Model file for the job. Use its own axes, mm. Round coordinates to 2 decimals unless told otherwise and drop trailing zeros. Use one line per item in the form item = value.
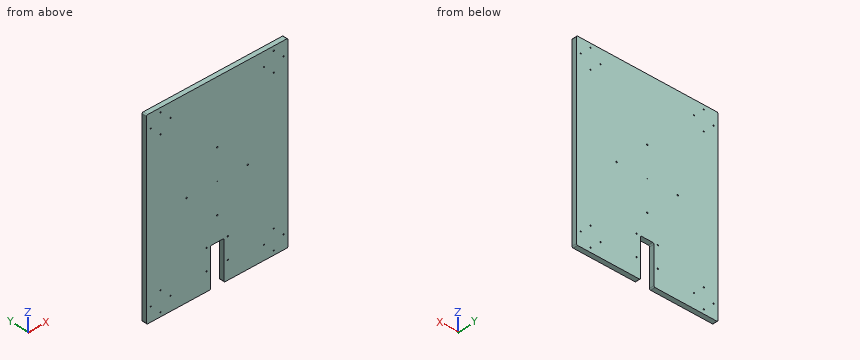
Autodesk Inventor part; units mm, degrees
ref_plane "YZ Plane" through (0, 0, 0) normal (1, 0, 0) x (0, 1, 0)
ref_plane "XZ Plane" through (0, 0, 0) normal (0, 1, 0) x (-1, 0, 0)
ref_plane "XY Plane" through (0, 0, 0) normal (0, 0, 1) x (1, 0, 0)
sketch "Sketch1" plane through (0, 0, 0) normal (0, 1, 0) x (-1, 0, 0)
  line L0 (300, 400) -> (-300, 400)
  line L1 (-300, 400) -> (-300, -400)
  line L2 (-300, -400) -> (300, -400)
  line L3 (300, -400) -> (300, 400)
  line L4 (300, 400) -> (-300, -400) construction
  circle A0 centre (130, 0) radius 3
  circle A1 centre (0, 130) radius 3
  circle A2 centre (-130, 0) radius 3
  circle A3 centre (0, -130) radius 3
  circle A4 centre (0, 0) radius 277.128
  line L5 (45, -232.128) -> (-45, -232.128)
  line L6 (-45, -232.128) -> (-45, -322.128)
  line L7 (-45, -322.128) -> (45, -322.128)
  line L8 (45, -322.128) -> (45, -232.128)
  line L9 (45, -232.128) -> (-45, -322.128) construction
  line L10 (-45, -232.128) -> (45, -322.128) construction
  circle A5 centre (45, -232.128) radius 2.5
  line L11 (28.5, -232.128) -> (-28.5, -232.128)
  line L12 (-28.5, -232.128) -> (-28.5, -322.128)
  line L13 (-28.5, -322.128) -> (28.5, -322.128)
  line L14 (28.5, -322.128) -> (28.5, -232.128)
  line L15 (28.5, -232.128) -> (-28.5, -322.128) construction
  line L16 (-28.5, -232.128) -> (28.5, -322.128) construction
  line L17 (45, -322.128) -> (-45, -322.128)
  line L18 (-45, -322.128) -> (-45, -400)
  line L19 (-45, -400) -> (45, -400)
  line L20 (45, -400) -> (45, -322.128)
  line L21 (28.5, -322.128) -> (-28.5, -322.128)
  line L22 (-28.5, -322.128) -> (-28.5, -400)
  line L23 (-28.5, -400) -> (28.5, -400)
  line L24 (28.5, -400) -> (28.5, -322.128)
  circle A6 centre (45, -322.128) radius 2.5
  circle A7 centre (-45, -232.128) radius 2.5
  circle A8 centre (-45, -322.128) radius 2.5
  circle A9 centre (0, 0) radius 1
  point P0 (0, -277.128)
  point P1 (28.5, -400)
  dimension "d10" = 554.256
  dimension "d0" = 600
  dimension "d1" = 800
  dimension "d2" = 6
  dimension "d3" = 130
  dimension "d6" = 360
  dimension "d41" = 90
  dimension "d42" = 90
  dimension "d43" = 5
  dimension "d52" = 57
  dimension "d75" = 90
  dimension "d78" = 90
  dimension "d82" = 2
extrude "Extrusion1" add sketch "Sketch1" along normal blind 20 contours L3 L2 L20 A6 L8 A4 L6 A8 L18 L1 L0 | L2 L24 L7 A6 L20 | L18 A8 L7 L22 L2 | L14 A4 L8 A6 L7 | L7 A8 L6 A4 L12 | L14 L5 A5 L8 A4 | A4 L6 A7 L5 L12 | A4 L8 A5 L5 A7 L6
sketch "Sketch3" plane through (0, 20, 0) normal (0, 1, 0) x (1, 0, 0)
  line L0 (-300, -400) -> (-180, -400)
  line L1 (-180, -400) -> (-180, -280)
  line L2 (-180, -280) -> (-300, -280)
  line L3 (-300, -280) -> (-300, -400)
  line L4 (-300, -400) -> (-180, -280) construction
  line L5 (-180, -400) -> (-300, -280) construction
  line L6 (-300, 400) -> (-300, -400)
  line L7 (-300, -400) -> (300, -400)
  circle A0 centre (-282, -340) radius 2.5
  circle A1 centre (-240, -382) radius 2.5
  circle A2 centre (-198, -340) radius 2.5
  circle A3 centre (-240, -298) radius 2.5
  line L8 (300, 400) -> (-300, 400)
  circle A4 centre (-240, 382) radius 2.5
  line L9 (-300, 400) -> (-300, 280)
  line L10 (-180, 280) -> (-300, 400) construction
  line L11 (-180, 280) -> (-180, 400)
  line L12 (-180, 400) -> (-300, 400)
  line L13 (-300, 280) -> (-180, 400) construction
  circle A5 centre (-198, 340) radius 2.5
  circle A6 centre (-282, 340) radius 2.5
  circle A7 centre (-240, 298) radius 2.5
  line L14 (-300, 280) -> (-180, 280)
  circle A8 centre (240, -298) radius 2.5
  line L15 (180, -280) -> (180, -400)
  line L16 (300, -400) -> (180, -280) construction
  line L17 (300, -400) -> (300, -280)
  line L18 (300, -280) -> (180, -280)
  line L19 (180, -400) -> (300, -280) construction
  circle A9 centre (282, -340) radius 2.5
  circle A10 centre (198, -340) radius 2.5
  circle A11 centre (240, -382) radius 2.5
  line L20 (180, -400) -> (300, -400)
  circle A12 centre (240, 382) radius 2.5
  line L21 (180, 400) -> (180, 280)
  line L22 (300, 280) -> (180, 400) construction
  line L23 (300, 280) -> (300, 400)
  line L24 (300, 400) -> (180, 400)
  line L25 (180, 280) -> (300, 400) construction
  circle A13 centre (282, 340) radius 2.5
  circle A14 centre (198, 340) radius 2.5
  circle A15 centre (240, 298) radius 2.5
  line L26 (180, 280) -> (300, 280)
  point P0 (0, 0)
  point P1 (-240, -340)
  point P2 (-240, 340)
  point P3 (240, -340)
  point P4 (240, 340)
  dimension "d53" = 120
  dimension "d54" = 120
  dimension "d55" = 60
  dimension "d56" = 60
  dimension "d57" = 5
  dimension "d58" = 42
  dimension "d61" = 360
  dimension "d67" = 680
  dimension "d70" = 480
extrude "Extrusion3" cut sketch "Sketch3" against normal through all contours A0 | A1 | A2 | A3 | A4 | A5 | A6 | A7 | A8 | A9 | A10 | A11 | A12 | A13 | A14 | A15
fillet "Fillet3" radius 5 8 edges at (300, 10, 400) (300, 10, -400) (-28.5, 10, -400) (28.5, 10, -400) (-28.5, 10, -232.128) (28.5, 10, -232.128) (-300, 10, -400) (-300, 10, 400)
equation "\"d0\" = Width"
equation "\"d1\" = Length"
equation "\"Width\" = 600"
equation "\"Length\" = 800"
equation "\"BearingHoleRadius1\" = 130"
properties part number "turntablebase"
1. Cut at A-A, the plane y = 3.75. Give the number of separate pieces and of enclosed holes in the cut face, plus the area to 3 significant figures.
Geometry check:
separate_pieces = 1
enclosed_holes = 25
area = 470,000 mm^2
2. Flat gauge pins, fed straight in: pin 1 (6.5 mm diameter, centred on x = 45, z = -232.128, fed in from -Y); pin 2 (2 mm diameter, centred on x = 1.5, y = 12.5, fed in from -Z). Where does each tip first touch, or does it go through?
Geometry check:
pin_1 = 0
pin_2 = -232.13
3. Wall check: probe 1 along Z at (x, y) = (282, 10.5); probe 2 along Z at (x, y) = (-240, 7); probe 3 along Z at (x, y) = (-45, 11.5). Give the ranges that are in metal, low to high.
Geometry check:
probe_1 = -400 to -342.5, -337.5 to 337.5, 342.5 to 400
probe_2 = -400 to -384.5, -379.5 to -300.5, -295.5 to 295.5, 300.5 to 379.5, 384.5 to 400
probe_3 = -400 to -324.63, -319.63 to -234.63, -229.63 to 400
